For this review, take the finished solid that the model builds, in its own axes (mm). Face numbers are marked on the shaded views. A direction names the side the tool comes from. Coordinates: 2 decimals unless noted, no trailing zeros. Order: outer loops, then holes, each group sorted by start corner. A loop starts at its lowest first (then second) coordinate and runs counter-clockwise, first axis right, second up. Notation, with made-up numbers: (5, 53) - (60, 53) arc R34 ccw to (60, 87) - close; hole circle Ø8 at (2.25, 43). An arc over 180 degrees is marked (long way). One line per item, written item: value. Start each with the question number.
(1) Consider section A-A on z = -7.62. Write out the cut boundary in (x, y) (3 decimals), then the cut area to 3 significant figures.
(2) For the marked faces 4, 5, 6 and 7, list the 3-axis set-ups (+Z, -Z, +X, -X, +Y, -Y) from which the entire face can be reached by the end or side of a thin tool; tool diameter is ignored.
(3) Consider section C-C on y = 30. Write out the cut boundary in (x, z) (3 decimals).
(4) Consider section B-B on x = 5. Write out the cut boundary in (y, z) (3 decimals).
(5) Clearance check with flat-ended pins moving along their axes: pin 1 (2.5 mm diameter, centred on y = 31, z = -20.5, fed in from -X); pin 2 (4 mm diameter, centred on x = 28, y = 26, fed in from +Z); pin 3 (2 mm diameter, centred on y = 31.5, z = 8, fed in from +X). State where each tip first meets the part, or that it passes through.
(6) To check wall thickness, follow line 1 along X through (y, z) = (5.25, -7.62) (3 decimals); line 2 along Z through (x, y) = (5, 27.25) (3 decimals); line 3 along Z through (x, y) = (41.5, 20). State the ranges of each line that lie inside material, in increasing order.
(7) Mouldability with a two-part tool opening along Z and no side actions: class the marked faces 1, 2 and 3 as released by +Z, released by -Z, zero draft, split by the parting line, or undercut.
(8) Consider section D-D on x = 23. Write out the cut boundary in (y, z).
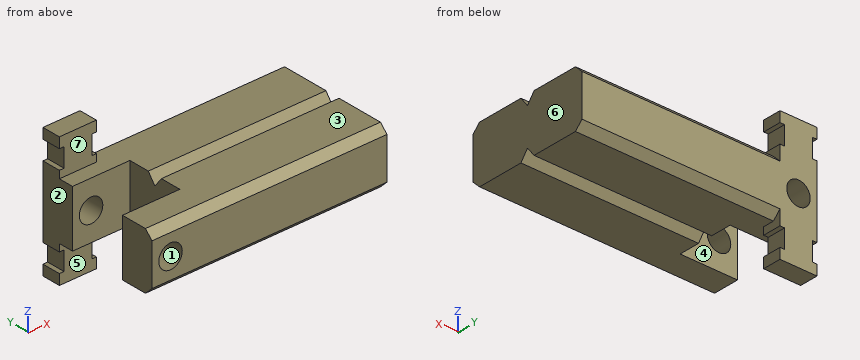
```python
from build123d import *

# Parameters (mm, degrees)
BOSS_EXTRUDE1_DEPTH = 63.5
CHAMFER1_SIZE       = 2
BOSS_EXTRUDE2_DEPTH = 5
SKETCH5_R           = 3.175
CUT_EXTRUDE3_DEPTH  = 76.963303483
SKETCH6_R           = 3.175
CUT_EXTRUDE4_DEPTH  = 7.62


with BuildPart() as part:
    # Sketch1 → Boss-Extrude1 (new body)
    with BuildSketch(Plane(origin=(0, 0, 0), x_dir=(0, 0, -1), z_dir=(1, 0, 0))):
        Polygon((0, 0), (15.24, 0), (15.24, 14.637), (12.62, 16.637), (15.24, 18.637), (15.24, 33.274), (0, 33.274), (0, 18.637), (2.62, 16.637), (0, 14.637), align=None)
    extrude(amount=BOSS_EXTRUDE1_DEPTH)

    # Chamfer1
    chamfer1_edges = [part.edges().sort_by_distance(p)[0] for p in [
        (31.75, 33.274, 0),
        (31.75, 33.274, -15.24),
        (31.75, 0, -15.24),
        (31.75, 0, 0),
    ]]
    chamfer(chamfer1_edges, length=CHAMFER1_SIZE)

    # Sketch4 → Boss-Extrude2 (add)
    with BuildSketch(Plane(origin=(0, 33.274, 0), x_dir=(1, 0, 0), z_dir=(0, 1, 0))):
        Polygon((10, 25.12), (0, 25.12), (0, 22.32), (1.25, 22.32), (1.25, 17.24), (0, 17.24), (0, -2), (1.25, -2), (1.25, -7.08), (0, -7.08), (0, -9.88), (10, -9.88), (10, -7.08), (8.75, -7.08), (8.75, -2), (10, -2), (10, 17.24), (8.75, 17.24), (8.75, 22.32), (10, 22.32), align=None)
    extrude(amount=-BOSS_EXTRUDE2_DEPTH)

    # Sketch5 → Cut-Extrude3 (cut, through all)
    with BuildSketch(Plane(origin=(0, 33.274, 0), x_dir=(1, 0, 0), z_dir=(0, 1, 0))):
        with Locations(Location((5, 7.62, 0), (0, 0, 270))):
            Circle(SKETCH5_R)
    extrude(amount=-CUT_EXTRUDE3_DEPTH, mode=Mode.SUBTRACT)

    # Sketch6 → Cut-Extrude4 (cut, symmetric)
    # profile 1 of 3: a face of its own
    with BuildSketch(Plane(origin=(0, 16.637, 0), x_dir=(-1, 0, 0), z_dir=(0, -1, 0))):
        with BuildLine():
            ThreePointArc((-15.5, 7.620000044), (-12.424621187, 15.044621218), (-5, 18.12))
            Line((-5, 18.12), (-15.5, 18.12))
            Line((-15.5, 18.12), (-15.5, 7.620000044))
        make_face()
    # profile 2 of 3: a face of its own
    with BuildSketch(Plane(origin=(0, 16.637, 0), x_dir=(-1, 0, 0), z_dir=(0, -1, 0))):
        with BuildLine():
            Line((5.5, 18.12), (-5, 18.12))
            ThreePointArc((-5, 18.12), (-12.424621187, 15.044621218), (-15.5, 7.620000044))
            ThreePointArc((-15.5, 7.620000044), (-12.424621218, 0.195378813), (-5, -2.88))
            Line((-5, -2.88), (5.5, -2.88))
            Line((5.5, -2.88), (5.5, 18.12))
        make_face()
        with Locations(Location((-5, 7.62, 0), (0, 0, 270))):
            Circle(SKETCH6_R, mode=Mode.SUBTRACT)
    # profile 3 of 3: a face of its own
    with BuildSketch(Plane(origin=(0, 16.637, 0), x_dir=(-1, 0, 0), z_dir=(0, -1, 0))):
        with BuildLine():
            ThreePointArc((-5, -2.88), (-12.424621218, 0.195378813), (-15.5, 7.620000044))
            Line((-15.5, 7.620000044), (-15.5, -2.88))
            Line((-15.5, -2.88), (-5, -2.88))
        make_face()
    extrude(amount=CUT_EXTRUDE4_DEPTH, both=True, mode=Mode.SUBTRACT)


solid = part.part
```
Geometry check:
1. outline: (0, 0) - (1.825, 0) - (1.825, 9.017) - (0, 9.017) - close; (0, 24.257) - (1.825, 24.257) - (1.825, 33.274) - (0, 33.274) - close; (8.175, 0) - (63.5, 0) - (63.5, 33.274) - (8.175, 33.274) - (8.175, 24.257) - (15.5, 24.257) - (15.5, 9.017) - (8.175, 9.017) - close
1. area: 1,760 mm^2
2. face 4: +Z, -Z, -X
2. face 5: -Z, +X, -X, -Y
2. face 6: +Z, -Z, +X, +Y, -Y
2. face 7: +Z, +X, -X, -Y
3. outline: (0, -25.12) - (10, -25.12) - (10, -22.32) - (8.75, -22.32) - (8.75, -17.24) - (10, -17.24) - (10, -15.24) - (63.5, -15.24) - (63.5, 0) - (10, 0) - (10, 2) - (8.75, 2) - (8.75, 7.08) - (10, 7.08) - (10, 9.88) - (0, 9.88) - (0, 7.08) - (1.25, 7.08) - (1.25, 2) - (0, 2) - (0, -17.24) - (1.25, -17.24) - (1.25, -22.32) - (0, -22.32) - close; hole circle Ø6.35 at (5, -7.62)
4. outline: (0, -13.24) - (2, -15.24) - (9.017, -15.24) - (9.017, -10.795) - (0, -10.795) - close; (0, -4.445) - (9.017, -4.445) - (9.017, 0) - (2, 0) - (0, -2) - close; (24.257, -15.24) - (28.274, -15.24) - (28.274, -25.12) - (33.274, -25.12) - (33.274, -10.795) - (24.257, -10.795) - close; (24.257, -4.445) - (33.274, -4.445) - (33.274, 9.88) - (28.274, 9.88) - (28.274, 0) - (24.257, 0) - close
5. pin 1: stops at x = 1.25
5. pin 2: stops at z = 0
5. pin 3: stops at x = 10
6. line 1: x = 0 to 1.825, 8.175 to 63.5
6. line 2: z = -15.24 to -10.795, -4.445 to 0
6. line 3: z = -15.24 to 0
7. face 1: undercut
7. face 2: zero draft
7. face 3: released by +Z
8. outline: (0, -13.24) - (2, -15.24) - (14.64, -15.24) - (16.64, -12.62) - (18.64, -15.24) - (31.27, -15.24) - (33.27, -13.24) - (33.27, -2) - (31.27, 0) - (18.64, 0) - (16.64, -2.62) - (14.64, 0) - (2, 0) - (0, -2) - close
